```python
from build123d import *

# Parameters (mm, degrees)
F0_W     = 40
F0_H     = 35
F1_DEPTH = 1.8
F3_DEPTH = 1.801
F5_DEPTH = 1.801
F6_R     = 3.365697
F7_DEPTH = 1.801


with BuildPart() as f1:
    # F0 (on Top) → F1 (new body)
    with BuildSketch(Plane.XY):
        Rectangle(F0_W, F0_H)
    extrude(amount=F1_DEPTH)

    # F2 (on face) → F3 (cut, through all)
    with BuildSketch(Plane.XY.offset(1.8)):
        Polygon((20, 17.5), (12.16623, 17.5), (20, -17.5), align=None)
    extrude(amount=-F3_DEPTH, mode=Mode.SUBTRACT)

    # F4 (on face) → F5 (cut, through all)
    with BuildSketch(Plane.XY.offset(1.8)):
        with BuildLine():
            ThreePointArc((-13.312635, -17.5), (-18.192213, -9.33692), (-20, 0))
            Line((-20, 0), (-20, -17.5))
            Line((-20, -17.5), (-13.312635, -17.5))
        make_face()
        with BuildLine():
            ThreePointArc((-20, 0.962044), (-18.408216, 9.713903), (-14.106414, 17.5))
            Line((-14.106414, 17.5), (-20, 17.5))
            Line((-20, 17.5), (-20, 0.962044))
        make_face()
    extrude(amount=-F5_DEPTH, mode=Mode.SUBTRACT)

    # F6 (on face) → F7 (cut, through all)
    with BuildSketch(Plane.XY.offset(1.8)):
        with Locations((10.903767, -9.809669)):
            Circle(F6_R)
    extrude(amount=-F7_DEPTH, mode=Mode.SUBTRACT)


solid = f1.part
```
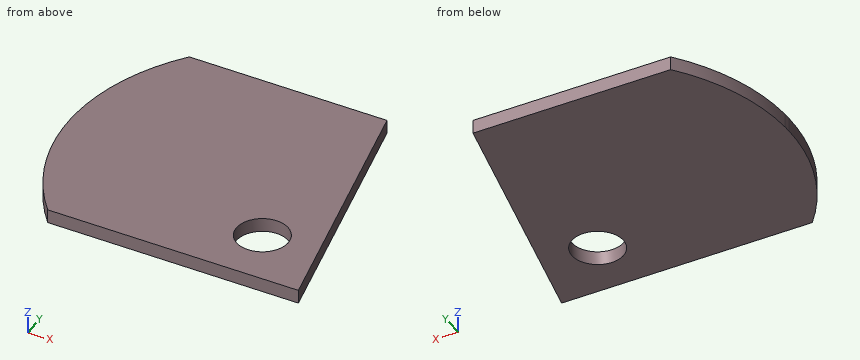
The listing builds one solid part. Answer for the finished solid, in the listing's coordinates (mm). Coordinates: 2 decimals unless noted, no trailing zeros. Write each loop counter-clockwise with the first axis right and the second up, starting at its lowest first coordinate (ties: lowest second). Pieces come first, ordered by that corner, then holes. Notation, with made-up numbers: (40.5, 23.25) - (89.5, 23.25) arc R23 cw to (89.5, 49.25) - close; hole circle Ø3 at (-14, 66). An arc over 180 degrees is marked (long way). Return JSON: item names as keys, results as strings. Group by question number.
1. A cutting plane is placed at A-A, the plane y = -12.5. Determine the outline of the cut face in (x, z).
2. A cutting plane is placed at C-C, the plane y = 4.5. Determine the outline of the cut face in (x, z).
3. Given pin 1 (1 mm diameter, centred on x = 11, y = 2, fed in from -Z), flat-ended and moving along its own axis, determine where the tip first touches the part or whether it passes through.
4. Straight lines are drawn through the part: L1, parallel to X at y = -11, z = 0.8; L2, parallel to Y at x = 10, z = 1; L3, parallel to X at y = -9.5, z = 1.55. For each, find the intervals that lie inside material, in ascending order.
5. A cutting plane is placed at B-B, the plane z = 1.45. Determine the outline of the cut face in (x, y), plus the area to 3 significant figures.
6. A cutting plane is placed at D-D, the plane y = -1.5. Determine the outline of the cut face in (x, z), plus the area to 3 significant figures.
Ans:
{
 "1": {"outline": "(-16.75, 0) - (8.88, 0) - (8.88, 1.8) - (-16.75, 1.8) - close; (12.93, 0) - (18.88, 0) - (18.88, 1.8) - (12.93, 1.8) - close"},
 "2": {"outline": "(-19.71, 0) - (15.08, 0) - (15.08, 1.8) - (-19.71, 1.8) - close"},
 "3": {"pin 1": "z = 0"},
 "4": {"L1": "-17.49 to 7.76, 14.05 to 18.55", "L2": "-17.5 to -13.05, -6.57 to 17.5", "L3": "-18.13 to 7.55, 14.26 to 18.21"},
 "5": {"outline": "(-20, 0) arc R27.5 ccw to (-13.31, -17.5) - (20, -17.5) - (12.17, 17.5) - (-14.11, 17.5) arc R27.5 ccw to (-20, 0.96) - close; hole circle Ø6.73 at (10.9, -9.81)", "area": "1,160 mm²"},
 "6": {"outline": "(-19.93, 0) - (16.42, 0) - (16.42, 1.8) - (-19.93, 1.8) - close", "area": "65.4 mm²"}
}
